For this review, take the finished solid that the model builds, in its own axes (mm). A direction names the side the tool comes from. Round coordinates to 2 decimals unless told otherwise and drop trailing zeros. Write each loop counter-clockwise with the first axis right and the second up, starting at its lowest first coordinate (ties: lowest second). Pieces come first, ordered by that corner, then holes. Notation, with made-up numbers: (54.5, 20.25) -> (113.5, 20.25) arc R23 ccw to (113.5, 32.25) -> close; hole circle Ø7 at (17.5, 87.25). An arc over 180 degrees is marked (long way). Answer in a Markdown table with one row per item.
from build123d import *

# Parameters (mm, degrees)
ESQUISSE1_W             = 55
ESQUISSE1_H             = 23
BOSS_EXTRU_1_DEPTH      = 5
ESQUISSE2_R             = 3
ENL_V_MAT_EXTRU_1_DEPTH = 5
ENL_V_MAT_EXTRU_2_DEPTH = 10
ESQUISSE5_W             = 5
ESQUISSE5_H             = 5
ESQUISSE5_W_2           = 35
ENL_V_MAT_EXTRU_3_DEPTH = 6
ESQUISSE7_W             = 5
ESQUISSE7_H             = 3
ENL_V_MAT_EXTRU_4_DEPTH = 6


with BuildPart() as part:
    # Esquisse1 → Boss.-Extru.1 (new body)
    with BuildSketch(Plane(origin=(0, 0, 0), x_dir=(1, 0, 0), z_dir=(0, 1, 0))):
        with Locations((0, 4)):
            Rectangle(ESQUISSE1_W, ESQUISSE1_H)
    extrude(amount=BOSS_EXTRU_1_DEPTH)

    # Esquisse2 → Enlèv. mat.-Extru.1 (cut)
    with BuildSketch(Plane(origin=(0, 5, 0), x_dir=(1, 0, 0), z_dir=(0, 1, 0))):
        with Locations((-22.5, 5)):
            Circle(ESQUISSE2_R)
        with Locations((22.5, 5)):
            Circle(ESQUISSE2_R)
    extrude(amount=-ENL_V_MAT_EXTRU_1_DEPTH, mode=Mode.SUBTRACT)

    # Esquisse4 → Enlèv. mat.-Extru.2 (cut)
    with BuildSketch(Plane(origin=(0, 5, 0), x_dir=(1, 0, 0), z_dir=(0, 1, 0))):
        Polygon((-15, 3.5), (-15, 1.75), (-16.5, 1.75), (-16.5, -1), (-15, -1), (-15, -2.5), (-12.25, -2.5), (-12.25, -1), (-10.75, -1), (-10.75, 1.75), (-12.25, 1.75), (-12.25, 3.5), align=None)
        Polygon((12.25, 3.5), (15, 3.5), (15, 1.75), (16.5, 1.75), (16.5, -1), (15, -1), (15, -2.5), (12.25, -2.5), (12.25, -1), (10.75, -1), (10.75, 1.75), (12.25, 1.75), align=None)
    extrude(amount=-ENL_V_MAT_EXTRU_2_DEPTH, mode=Mode.SUBTRACT)

    # Esquisse5 → Enlèv. mat.-Extru.3 (cut, through all)
    with BuildSketch(Plane(origin=(0, 5, 0), x_dir=(1, 0, 0), z_dir=(0, 1, 0))):
        with Locations((-25, -5)):
            Rectangle(ESQUISSE5_W, ESQUISSE5_H)
        with Locations((0, -5)):
            Rectangle(ESQUISSE5_W_2, ESQUISSE5_H)
        with Locations((25, -5)):
            Rectangle(ESQUISSE5_W, ESQUISSE5_H)
    extrude(amount=-ENL_V_MAT_EXTRU_3_DEPTH, mode=Mode.SUBTRACT)

    # Esquisse7 → Enlèv. mat.-Extru.4 (cut, through all)
    with BuildSketch(Plane(origin=(0, 5, 0), x_dir=(1, 0, 0), z_dir=(0, 1, 0))):
        with Locations((0, 14)):
            Rectangle(ESQUISSE7_W, ESQUISSE7_H)
        with Locations((10, 14)):
            Rectangle(ESQUISSE7_W, ESQUISSE7_H)
        with Locations((-10, 14)):
            Rectangle(ESQUISSE7_W, ESQUISSE7_H)
    extrude(amount=-ENL_V_MAT_EXTRU_4_DEPTH, mode=Mode.SUBTRACT)


solid = part.part
1) Consider section C-C on z = -13.75. State the section outline as (x, y) points.
Solved:
| item | result |
|---|---|
| outline | (-27.5, 0) -> (-12.5, 0) -> (-12.5, 5) -> (-27.5, 5) -> close; (-7.5, 0) -> (-2.5, 0) -> (-2.5, 5) -> (-7.5, 5) -> close; (2.5, 0) -> (7.5, 0) -> (7.5, 5) -> (2.5, 5) -> close; (12.5, 0) -> (27.5, 0) -> (27.5, 5) -> (12.5, 5) -> close |
2) For line 1 (X direction, y = 3.15, z = -13.5); line 2 (X direction, y = 0.9, z = 2.25); line 3 (X direction, y = 3, z = -5), list the stretches that pass through material, from the lowest coordinate up. Write a range as [from, to].
Solved:
| item | result |
|---|---|
| line 1 | [-27.5, -12.5], [-7.5, -2.5], [2.5, 7.5], [12.5, 27.5] |
| line 2 | [-27.5, -15], [-12.25, 12.25], [15, 27.5] |
| line 3 | [-27.5, -25.5], [-19.5, 19.5], [25.5, 27.5] |
3) Consider section B-B on z = 4.25. State the section outline as (x, y) points.
Solved:
| item | result |
|---|---|
| outline | (-22.5, 0) -> (-17.5, 0) -> (-17.5, 5) -> (-22.5, 5) -> close; (17.5, 0) -> (22.5, 0) -> (22.5, 5) -> (17.5, 5) -> close |
4) Mouldability with a two-part tool opening along X and no side actions: class faces 6 (the flat face through (-27.5, 2, -6)), 7 (the flat face through (-16.5, 3, 0)), 8 (the flat face through (16, 3, 1)), 9 (the flat face through (-5, 2, -15.5)) as pulls with the +X half, pulls with the -X half, needs draft (parallel to the pull), parting line crosses it, or undercut.
Solved:
| item | result |
|---|---|
| face 6 | pulls with the -X half |
| face 7 | undercut |
| face 8 | undercut |
| face 9 | needs draft |
5) Consider section A-A on z = -5. State the section outline as (x, y) points.
Solved:
| item | result |
|---|---|
| outline | (-27.5, 0) -> (-25.5, 0) -> (-25.5, 5) -> (-27.5, 5) -> close; (-19.5, 0) -> (19.5, 0) -> (19.5, 5) -> (-19.5, 5) -> close; (25.5, 0) -> (27.5, 0) -> (27.5, 5) -> (25.5, 5) -> close |
6) Consider section D-D on x = -9. State the section outline as (y, z) points, then the cut area to 3 significant figures.
Solved:
| item | result |
|---|---|
| outline | (0, -12.5) -> (5, -12.5) -> (5, 2.5) -> (0, 2.5) -> close |
| area | 75.0 mm² |
7) For faces 1 (the flat face through (27.5, 2, -6)), 2 (the flat face through (16.5, 3, 0)), 3 (the flat face through (2.5, 3, -14)), 4 (the flat face through (0, 5, -7)), 5 (the flat face through (14, 3, -3.5)), list the 3-axis set-ups (+Z, -Z, +X, -X, +Y, -Y) from which the entire face can be reached by the end or side of a thin tool; tool diameter is ignored.
Solved:
| item | result |
|---|---|
| face 1 | +Z, -Z, +X, +Y, -Y |
| face 2 | +Y, -Y |
| face 3 | -Z, +Y, -Y |
| face 4 | +Z, -Z, +X, -X, +Y |
| face 5 | +Z, +Y, -Y |
8) Clearance check with flat-ended pins moving along their axes: pin 1 Ø2.5 at (x, y) = (24, 3) entering from +Z; pin 2 Ø1.2 at (x, y) = (11, 3) entering from -Z; pin 3 Ø0.8 at (x, y) = (14.5, 2) entering from +Z. State where each tip first meets the part, or that it passes through.
Solved:
| item | result |
|---|---|
| pin 1 | z = 2.5 |
| pin 2 | z = -12.5 |
| pin 3 | z = -3.5 |
